```python
from build123d import *

# Parameters (mm, degrees)
SKETCH_1_R          = 50
SKETCH_1_R_2        = 15
SKETCH_1_R_3        = 2.15
EXTRUDE_1_DEPTH     = 3
SKETCH_2_R          = 2.15
CUT_EXTRUDE_1_DEPTH = 3
CUT_EXTRUDE_2_DEPTH = 3


with BuildPart() as part:
    # 草图1 → 凸台-拉伸1 (new body)
    with BuildSketch(Plane.XY):
        with Locations((-43.046732458, 46.816740082)):
            Circle(SKETCH_1_R)
        with Locations((-43.046732458, 46.816740082)):
            Circle(SKETCH_1_R_2, mode=Mode.SUBTRACT)
        with Locations((-58.927913307, 58.761439339)):
            Circle(SKETCH_1_R_3, mode=Mode.SUBTRACT)
        with Locations((-45.401306439, 26.870517329)):
            Circle(SKETCH_1_R_3, mode=Mode.SUBTRACT)
        with Locations((-24.546261263, 54.530363509)):
            Circle(SKETCH_1_R_3, mode=Mode.SUBTRACT)
    extrude(amount=EXTRUDE_1_DEPTH)

    # 草图2 → 切除-拉伸1 (cut)
    with BuildSketch(Plane(origin=(0, 0, 0), x_dir=(-1, 0, 0), z_dir=(0, 0, -1))):
        with Locations((11.795724887, 79.184319745)):
            Circle(SKETCH_2_R)
        with Locations((74.121262453, 79.184319745)):
            Circle(SKETCH_2_R)
        with Locations((74.121262453, 14.25722704)):
            Circle(SKETCH_2_R)
        with Locations((11.795724887, 14.25722704)):
            Circle(SKETCH_2_R)
    extrude(amount=-CUT_EXTRUDE_1_DEPTH, mode=Mode.SUBTRACT)

    # 草图3 → 切除-拉伸2 (cut)
    with BuildSketch(Plane(origin=(0, 0, 0), x_dir=(-1, 0, 0), z_dir=(0, 0, -1))):
        with BuildLine():
            Line((25.153451443, 60.790750239), (13.742198917, 69.103210849))
            ThreePointArc((13.742198917, 69.103210849), (12.525075816, 71.213815689), (13.27574755, 73.531688287))
            ThreePointArc((13.27574755, 73.531688287), (37.655506434, 86.451758462), (64.600480937, 80.512970235))
            ThreePointArc((64.600480937, 80.512970235), (65.932157971, 78.540792241), (65.408806124, 76.219380472))
            Line((65.408806124, 76.219380472), (57.141381217, 64.869952453))
            ThreePointArc((57.141381217, 64.869952453), (55.325889869, 63.698864431), (53.194378054, 64.05116171))
            ThreePointArc((53.194378054, 64.05116171), (40.603919689, 66.666996145), (29.023333751, 61.076623977))
            ThreePointArc((29.023333751, 61.076623977), (27.140836024, 60.223758694), (25.153451443, 60.790750239))
        make_face()
        with BuildLine():
            Line((20.364867546, 49.996457779), (6.402262109, 51.481543763))
            ThreePointArc((6.402262109, 51.481543763), (4.130184621, 50.774073872), (3.088066895, 48.634718735))
            ThreePointArc((3.088066895, 48.634718735), (11.417412674, 22.330292198), (34.796401106, 7.676836753))
            ThreePointArc((34.796401106, 7.676836753), (37.179073525, 8.185672261), (38.398349384, 10.295034206))
            Line((38.398349384, 10.295034206), (39.891525177, 24.333699088))
            ThreePointArc((39.891525177, 24.333699088), (39.388861968, 26.338320394), (37.709010103, 27.542178607))
            ThreePointArc((37.709010103, 27.542178607), (27.07731282, 34.776074136), (23.047462711, 46.987648143))
            ThreePointArc((23.047462711, 46.987648143), (22.286805197, 49.009740163), (20.364867546, 49.996457779))
        make_face()
        with BuildLine():
            Line((64.095220754, 55.325770919), (76.999649074, 61.051975191))
            ThreePointArc((76.999649074, 61.051975191), (79.436048033, 61.050732296), (81.068048719, 59.241695206))
            ThreePointArc((81.068048719, 59.241695206), (80.067278266, 31.668169586), (61.451649543, 11.302531276))
            ThreePointArc((61.451649543, 11.302531276), (59.077854783, 11.135354132), (57.329129141, 12.749296011))
            Line((57.329129141, 12.749296011), (51.633948612, 25.583810014))
            ThreePointArc((51.633948612, 25.583810014), (51.527502308, 27.741615653), (52.898356609, 29.411410393))
            ThreePointArc((52.898356609, 29.411410393), (61.458964865, 39.007149965), (62.40785352, 51.831417662))
            ThreePointArc((62.40785352, 51.831417662), (62.610499382, 53.888141158), (64.095220754, 55.325770919))
        make_face()
    extrude(amount=-CUT_EXTRUDE_2_DEPTH, mode=Mode.SUBTRACT)


solid = part.part
```
The model under review builds one solid part; all positions refer to its coordinate system, in mm. Round coordinates to 2 decimals unless told otherwise and drop trailing zeros. Order: outer loops, then holes, each group sorted by start corner. A loop starts at its lowest first (then second) coordinate and runs counter-clockwise, first axis right, second up.
(1) Mouldability with a two-part tool opening along X and no side actions: class faces 1 (the face through (-55.356, 63.705, 1.479)), 2 (the face through (-79.9, 80.61, 1.48)), 3 (the face through (-59.11, 11.124, 1.479)), 4 (the face through (-33, 59, 0)) as released by +X, released by -X, zero draft, split by the parting line, or undercut.
Working result:
face 1: undercut
face 2: split by the parting line
face 3: undercut
face 4: zero draft
(2) Take a section at A-A, the plane y = 37. State the section outline as (x, z) points, plus the area to 3 significant figures.
Working result:
outline: (-92.07, 0) - (-81.82, 0) - (-81.82, 3) - (-92.07, 3) - close; (-60.47, 0) - (-54.39, 0) - (-54.39, 3) - (-60.47, 3) - close; (-31.71, 0) - (-25.62, 0) - (-25.62, 3) - (-31.71, 3) - close; (-4.27, 0) - (5.98, 0) - (5.98, 3) - (-4.27, 3) - close
area: 98.0 mm2
(3) Take a section at B-B, the plane z = 1.9. Count the separate pieces of the cut face and the enclosed holes in it, plus the area to 3 significant figures.
Working result:
separate pieces: 1
enclosed holes: 11
area: 4,240 mm2
(4) For P1, Ø1.5, axis at y = 49, z = 1.5, coming from the +X side; P2, Ø1.5, axis at x = -76, z = 1, coming from the -Y side, all flat-tipped, find the tip position at first contact; note any pin that passes through.
Working result:
P1: stops at x = 6.93
P2: stops at y = 8.57
(5) Wall thickness on L1, parallel to X at y = 15, z = 1.25; L2, parallel to X at y = 78, z = 2; L3, parallel to X at y = 31, z = 2.4: over which ranges is each line inside the solid? List them lowest first.
Working result:
L1: x = -81.62 to -76.14, -72.1 to -67.29, -56.33 to -38.9, -18.8 to -13.81, -9.78 to -4.48
L2: x = -82.13 to -75.92, -72.33 to -65.98, -17.99 to -13.59, -10 to -3.96
L3: x = -90.48 to -79.79, -55.29 to -30.81, -6.31 to 4.39
(6) Take a section at C-C, the plane y = 71. State the section outline as (x, z) points, plus the area to 3 significant figures.
Working result:
outline: (-86.81, 0) - (-61.61, 0) - (-61.61, 3) - (-86.81, 3) - close; (-12.56, 0) - (0.72, 0) - (0.72, 3) - (-12.56, 3) - close
area: 115 mm2
